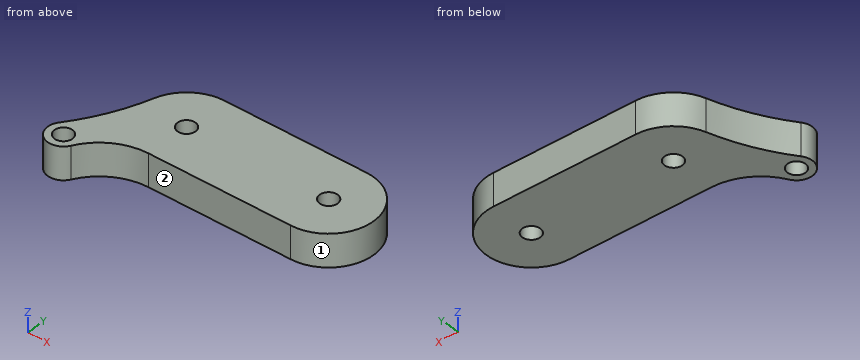
```python
from build123d import *

# Parameters (mm, degrees)
SKETCH1_R           = 1
BOSS_EXTRUDE1_DEPTH = 3.6


with BuildPart() as part:
    # Sketch1 → Boss-Extrude1 (new body)
    with BuildSketch(Plane.XY):
        with BuildLine():
            Line((0, 5), (16, 5))
            ThreePointArc((16, 5), (21, 0), (16, -5))
            Line((16, -5), (0, -5))
            ThreePointArc((0, -5), (-3.368878467, -5.934437461), (-5.775069682, -8.470725956))
            ThreePointArc((-5.775069682, -8.470725956), (-8.265817764, -9.127128459), (-8.725078251, -6.592612716))
            ThreePointArc((-8.725078251, -6.592612716), (-6.399016419, -2.812300799), (-4.818388045, 1.335341397))
            ThreePointArc((-4.818388045, 1.335341397), (-3.026821189, 3.979742893), (0, 5))
        make_face()
        with Locations((-7.323866259, -7.647577093)):
            Circle(SKETCH1_R, mode=Mode.SUBTRACT)
        Circle(SKETCH1_R, mode=Mode.SUBTRACT)
        with Locations((16, 0)):
            Circle(SKETCH1_R, mode=Mode.SUBTRACT)
    extrude(amount=BOSS_EXTRUDE1_DEPTH)


solid = part.part
```
The model under review builds one solid part; all positions refer to its coordinate system, in mm. Face numbers are marked on the shaded views. A direction names the side the tool comes from. Round coordinates to 2 decimals unless told otherwise and drop trailing zeros. Loops run counter-clockwise (first coordinate to the right, second up) from the corner with the lowest first, then second, coordinate; pieces in that order, holes last. Notation, with made-up numbers: (-5.75, 58) -> (11.25, 58) arc R14 ccw to (11.25, 69) -> close; hole circle Ø3 at (5.25, 33). An arc over 180 degrees is marked (long way). Answer in a Markdown table with one row per item.
1) Consider section D-D, the plane y = 3. Write out the cut boundary in (x, z).
Taken from the geometry:
| item | result |
|---|---|
| outline | (-4, 0) -> (20, 0) -> (20, 3.6) -> (-4, 3.6) -> close |
2) Wall thickness on line 1 along Y through (x, z) = (16, 0.85); line 2 along X through (y, z) = (-0.5, 0.8); line 3 along X through (y, z) = (0.25, 0.6): over which ranges is each line inside the solid? List them lowest first.
Taken from the geometry:
| item | result |
|---|---|
| line 1 | y = -5 to -1, 1 to 5 |
| line 2 | x = -5.41 to -0.87, 0.87 to 15.13, 16.87 to 20.97 |
| line 3 | x = -5.15 to -0.97, 0.97 to 15.03, 16.97 to 20.99 |
3) For pin 1 Ø2 at (y, z) = (-3, 1.5) entering from +X; pin 2 Ø2 at (y, z) = (-6, 2.5) entering from -X; pin 3 Ø1.8 at (x, z) = (10, 2) entering from -Y, all flat-tipped, find the tip position at first contact; note any pin that passes through.
Taken from the geometry:
| item | result |
|---|---|
| pin 1 | stops at x = 20.58 |
| pin 2 | stops at x = -8.95 |
| pin 3 | stops at y = -5 |
4) Consider section B-B, the plane z = 2.3. Write out the cut boundary in (x, y).
Taken from the geometry:
| item | result |
|---|---|
| outline | (-8.73, -6.59) arc R1.75 ccw (long way) to (-5.78, -8.47) arc R6.54 cw to (0, -5) -> (16, -5) arc R5 ccw to (16, 5) -> (0, 5) arc R5 ccw to (-4.82, 1.34) arc R23.71 cw to start; hole circle Ø2 at (-7.32, -7.65); hole circle Ø2 at (0, 0); hole circle Ø2 at (16, 0) |
5) Tool access review of the marked faces 1 and 2: name each direction out of +Z, -Z, +X, -X, +Y, -Y from which nothing blocks a thin tool from reaching the whole face with its end or side.
Taken from the geometry:
| item | result |
|---|---|
| face 1 | +Z, -Z, +X |
| face 2 | +Z, -Z, +X, -Y |
6) Consider section C-C, the plane y = 0. Write out the cut boundary in (x, z), plus the area to 3 significant figures.
Taken from the geometry:
| item | result |
|---|---|
| outline | (-5.23, 0) -> (-1, 0) -> (-1, 3.6) -> (-5.23, 3.6) -> close; (1, 0) -> (15, 0) -> (15, 3.6) -> (1, 3.6) -> close; (17, 0) -> (21, 0) -> (21, 3.6) -> (17, 3.6) -> close |
| area | 80.0 mm² |
7) Consider section A-A, the plane x = -7. Write out the cut boundary in (y, z).
Taken from the geometry:
| item | result |
|---|---|
| outline | (-9.37, 0) -> (-8.59, 0) -> (-8.59, 3.6) -> (-9.37, 3.6) -> close; (-6.7, 0) -> (-3.95, 0) -> (-3.95, 3.6) -> (-6.7, 3.6) -> close |
